from build123d import *

# Parameters (mm, degrees)
SKETCH1_R           = 14.2875
BOSS_EXTRUDE1_DEPTH = 6.35
SKETCH2_R           = 15.08125
BOSS_EXTRUDE2_DEPTH = 1.5748


with BuildPart() as part:
    # Sketch1 → Boss-Extrude1 (new body)
    with BuildSketch(Plane.XY):
        Circle(SKETCH1_R)
        Polygon((6.35, 3.666174209), (0, 7.332348419), (-6.35, 3.666174209), (-6.35, -3.666174209), (0, -7.332348419), (6.35, -3.666174209), align=None, mode=Mode.SUBTRACT)
    extrude(amount=BOSS_EXTRUDE1_DEPTH)

    # Sketch2 → Boss-Extrude2 (add)
    with BuildSketch(Plane(origin=(0, 0, 0), x_dir=(-1, 0, 0), z_dir=(0, 0, -1))):
        Circle(SKETCH2_R)
        Polygon((0, 7.332348419), (-6.35, 3.666174209), (-6.35, -3.666174209), (0, -7.332348419), (6.35, -3.666174209), (6.35, 3.666174209), align=None, mode=Mode.SUBTRACT)
    extrude(amount=BOSS_EXTRUDE2_DEPTH)


solid = part.part
Build history of the part. All positions in model axes, mm. A direction names the side the tool comes from. Give positions to 0.01 mm unless a question says otherwise; leave off trailing zeros. Order: outer loops, then holes, each group sorted by start corner. A loop starts at its lowest first (then second) coordinate and runs counter-clockwise, first axis right, second up. Notation, with made-up numbers: M -7.75,60.25 L 30.25,60.25 A34 cw 30.25,97.25 Z; hole C 54,61 d7. An arc over 180 degrees is marked long. Use one line per item in the form item = value.
Q1. Wall check: probe 1 along Y at (x, z) = (5, -0.75); probe 2 along Y at (x, z) = (-5.5, 1.5); probe 3 along X at (y, z) = (2.5, 4). Give the ranges that are in metal, low to high.
Conclusion:
probe_1 = -14.23 to -4.45, 4.45 to 14.23
probe_2 = -13.19 to -4.16, 4.16 to 13.19
probe_3 = -14.07 to -6.35, 6.35 to 14.07
Q2. Slice it at C-C, the plane x = -2. Write the cut outline in (y, z), and give its area (3 significant figures).
Conclusion:
outline = M -14.95,-1.57 L -6.18,-1.57 L -6.18,6.35 L -14.15,6.35 L -14.15,0 L -14.95,0 Z; M 6.18,-1.57 L 14.95,-1.57 L 14.95,0 L 14.15,0 L 14.15,6.35 L 6.18,6.35 Z
area = 129 mm2
Q3. Slice it at D-D, the plane y = -10. Write the cut outline in (x, z).
Conclusion:
outline = M -11.29,-1.57 L 11.29,-1.57 L 11.29,0 L 10.2,0 L 10.2,6.35 L -10.2,6.35 L -10.2,0 L -11.29,0 Z
Q4. Which spindle directions (+Z, -Z, +X, -X, +Y, -Y) get a long thin tool onto all of the face, cutting with end or side? Do faces 4 (the flat face through (-7.75, -12.22, 0)), 5 (the flat face through (-6.35, 0, 2)), 6 (the flat face through (-7, 0, 6.35)). Say none if no direction does.
Conclusion:
face_4 = +Z
face_5 = +Z, -Z
face_6 = +Z, +X, -X, +Y, -Y
Q5. Slice it at B-B, the plane y = 0. Write the cut outline in (x, z), and give its area (3 significant figures).
Conclusion:
outline = M -15.08,-1.57 L -6.35,-1.57 L -6.35,6.35 L -14.29,6.35 L -14.29,0 L -15.08,0 Z; M 6.35,-1.57 L 15.08,-1.57 L 15.08,0 L 14.29,0 L 14.29,6.35 L 6.35,6.35 Z
area = 128 mm2
Q6. Pin check, flat tips, straight feed: P1, Ø1.5, axis at y = 1.5, z = 4.5, coming from the +X side; P2, Ø3, axis at x = -6, z = -0.5, coming from the +Y side; P3, Ø1, axis at x = 7.5, z = 1.5, coming from the -Y side. Stop position of each tip, or through.
Conclusion:
P1 = 14.27
P2 = 14.39
P3 = -12.46
Q7. Pull direction Y, two halves, no side cores. Call faces 1 (the flat face through (3.219, -5.474, 2.443)), 2 (the cylindrical face through (15.067, 0.663, -0.776)), 3 (the flat face through (-6.5, 0.2, -1.575)): released by +Y, released by -Y, zero draft, split by the parting line, or undercut.
Conclusion:
face_1 = undercut
face_2 = split by the parting line
face_3 = zero draft
